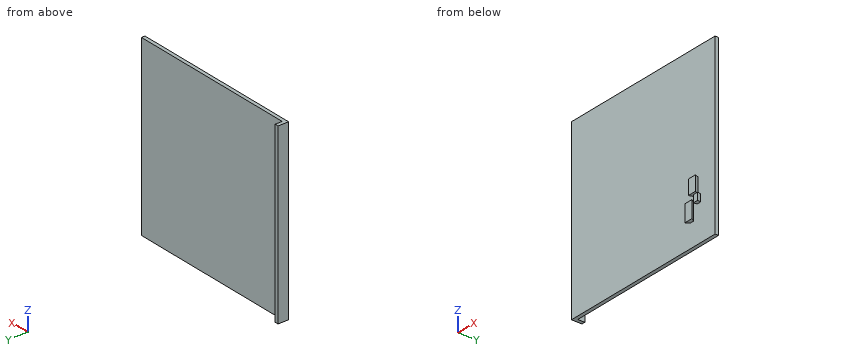
```python
from build123d import *

# Parameters (mm, degrees)
SKETCH1_W           = 500
SKETCH1_H           = 500
BOSS_EXTRUDE1_DEPTH = 10
SKETCH2_W           = 10
SKETCH2_H           = 500
BOSS_EXTRUDE2_DEPTH = 20
SKETCH3_W           = 24.824794579
SKETCH3_H           = 41.535737198
SKETCH3_H_2         = 47.922361064
SKETCH3_W_2         = 15.07825301
SKETCH3_H_3         = 20.670620926
BOSS_EXTRUDE3_DEPTH = 10
CUT_EXTRUDE4_DEPTH  = 50
CUT_EXTRUDE5_DEPTH  = 50
CUT_EXTRUDE6_DEPTH  = 22


with BuildPart() as part:
    # Sketch1 → Boss-Extrude1 (new body)
    with BuildSketch(Plane(origin=(0, 0, 0), x_dir=(1, 0, 0), z_dir=(0, 1, 0))):
        Rectangle(SKETCH1_W, SKETCH1_H)
    extrude(amount=BOSS_EXTRUDE1_DEPTH)

    # Sketch2 → Boss-Extrude2 (add)
    with BuildSketch(Plane(origin=(0, 10, 0), x_dir=(1, 0, 0), z_dir=(0, 1, 0))):
        with Locations((-245, 0)):
            Rectangle(SKETCH2_W, SKETCH2_H)
    extrude(amount=BOSS_EXTRUDE2_DEPTH)

    # Sketch3 → Boss-Extrude3 (add)
    with BuildSketch(Plane.XZ):
        with Locations((181.563787456, -100.472088386)):
            Rectangle(SKETCH3_W, SKETCH3_H)
        with Locations((169.151390168, -160.909121908)):
            Rectangle(SKETCH3_W, SKETCH3_H_2)
        with Locations((193.976184746, -136.947941376)):
            Rectangle(SKETCH3_W_2, SKETCH3_H_3)
    extrude(amount=BOSS_EXTRUDE3_DEPTH)

    # Sketch6 → Cut-Extrude4 (cut)
    with BuildSketch(Plane(origin=(0, 0, -184.87030244), x_dir=(-1, 0, 0), z_dir=(0, 0, -1))):
        Polygon((-156.738992878, -10), (-162.512495569, 0), (-156.738992878, 0), align=None)
        Polygon((-175.790284765, 0), (-181.563787457, 0), (-181.563787457, -10), align=None)
    extrude(amount=-CUT_EXTRUDE4_DEPTH, mode=Mode.SUBTRACT)

    # Sketch5 → Cut-Extrude5 (cut)
    with BuildSketch(Plane(origin=(0, 0, -121.239956985), x_dir=(-1, 0, 0), z_dir=(0, 0, -1))):
        Polygon((-172.79109251, 0), (-169.151390167, -10), (-169.151390167, 0), align=None)
        Polygon((-193.976184746, -10), (-190.336482403, 0), (-193.976184746, 0), align=None)
    extrude(amount=-CUT_EXTRUDE5_DEPTH, mode=Mode.SUBTRACT)

    # Sketch4 → Cut-Extrude6 (cut)
    with BuildSketch(Plane(origin=(0, 0, -147.283251839), x_dir=(-1, 0, 0), z_dir=(0, 0, -1))):
        Polygon((-186.437058241, -10), (-188.200328049, 0), (-186.437058241, 0), align=None)
        Polygon((-199.752041444, 0), (-201.515311251, 0), (-201.515311251, -10), align=None)
    extrude(amount=-CUT_EXTRUDE6_DEPTH, mode=Mode.SUBTRACT)


solid = part.part
```
Check sheet for the modelled part. Datum: model origin and axes. Units: mm. Round coordinates to 2 decimals unless told otherwise and drop trailing zeros. Loops run counter-clockwise (first coordinate to the right, second up) from the corner with the lowest first, then second, coordinate; pieces in that order, holes last. Notation, with made-up numbers: (-13, 36) -> (35, 36) arc R19 cw to (35, 46) -> close; hole circle Ø3 at (37, 82). An arc over 180 degrees is marked (long way). Answer in a Markdown table with one row per item.
Q1. Thickness scan on L1, parallel to Y at x = 196, z = -145.5; L2, parallel to Y at x = -111, z = -96.5; L3, parallel to X at y = 10.5, z = -90.5. Record the ranges inside material, lowest first.
Data:
| item | result |
|---|---|
| L1 | y = -10 to 10 |
| L2 | y = 0 to 10 |
| L3 | x = -250 to -240 |
Q2. Sectioned sample at A-A on z = 163. Enter the section's corners in (x, y).
Data:
| item | result |
|---|---|
| outline | (-250, 0) -> (250, 0) -> (250, 10) -> (-240, 10) -> (-240, 30) -> (-250, 30) -> close |
Q3. Sectioned sample at B-B on x = -155. Enter the section's corners in (y, z).
Data:
| item | result |
|---|---|
| outline | (0, -250) -> (10, -250) -> (10, 250) -> (0, 250) -> close |
Q4. Go/stop test with flat-tipped pins: P1, Ø11, axis at x = 170, y = -7.5, coming from the -Z side; P2, Ø4, axis at x = -195, z = -157.5, coming from the +Y side; P3, Ø10, axis at x = 91.5, z = 51.5, coming from the -Y side. Record where each tip stops, or that it passes through.
Data:
| item | result |
|---|---|
| P1 | stops at z = -184.87 |
| P2 | stops at y = 10 |
| P3 | stops at y = 0 |
Q5. Sectioned sample at C-C on y = 22. Enter the section's corners in (x, z), then the cut area to 3 significant figures.
Data:
| item | result |
|---|---|
| outline | (-250, -250) -> (-240, -250) -> (-240, 250) -> (-250, 250) -> close |
| area | 5,000 mm^2 |
